Input: dimensioned drawing with shaded views. Units: mm. Origin: part minimum x, y, z. Coordinates: 2 decimals unless noted, no trailing zeros. Order: outer loops, then holes, each group sorted by start corner. A loop starts at its lowest first (then second) coordinate and runs counter-clockwise, first axis right, second up. Notation, with made-up numbers: (21.25, -26) - (47.25, -26) arc R14 ccw to (47.25, -13) - close; hole circle Ø5 at (66.5, 20). An arc over 180 degrees is marked (long way). Answer as CSV lines item,"result". Start each with the question number.
Item 1: Draft query along Y for the marked faces 1, 2 and 3. Return one class per face: +Y half, -Y half, draft (parallel to the pull), parting line (faces both ways), or undercut.
Item 2: First-contact query: pin 1 (1.5 mm diameter, centred on y = 143.5, z = 11.5, fed in from +X); pin 2 (12 mm diameter, centred on x = 36.5, y = 100.5, fed in from +Z); pin 3 (1.5 mm diameter, centred on x = 12.5, z = 12, fed in from -Y). Flat tips, straight axial feed; report the tip coordinate or a pass-through.
Item 3: Section D-D (y = 98). Output: boundary loops of the cut face in (x, z).
Item 4: Section A-A (x = 30). Output: boundary loops of the cut face in (y, z), and give its area (3 significant figures).
Item 5: Section C-C (x = 12.5). Output: boundary loops of the cut face in (y, z).
Item 6: Section B-B (y = 142). Output: boundary loops of the cut face in (x, z).
Item 7: Material intervals for line 1 along X through (y, z) = (142, 5.5); line 2 along Y through (x, z) = (30, 9.5); line 3 along Z through (x, y) = (43, 84), sorted ascending.
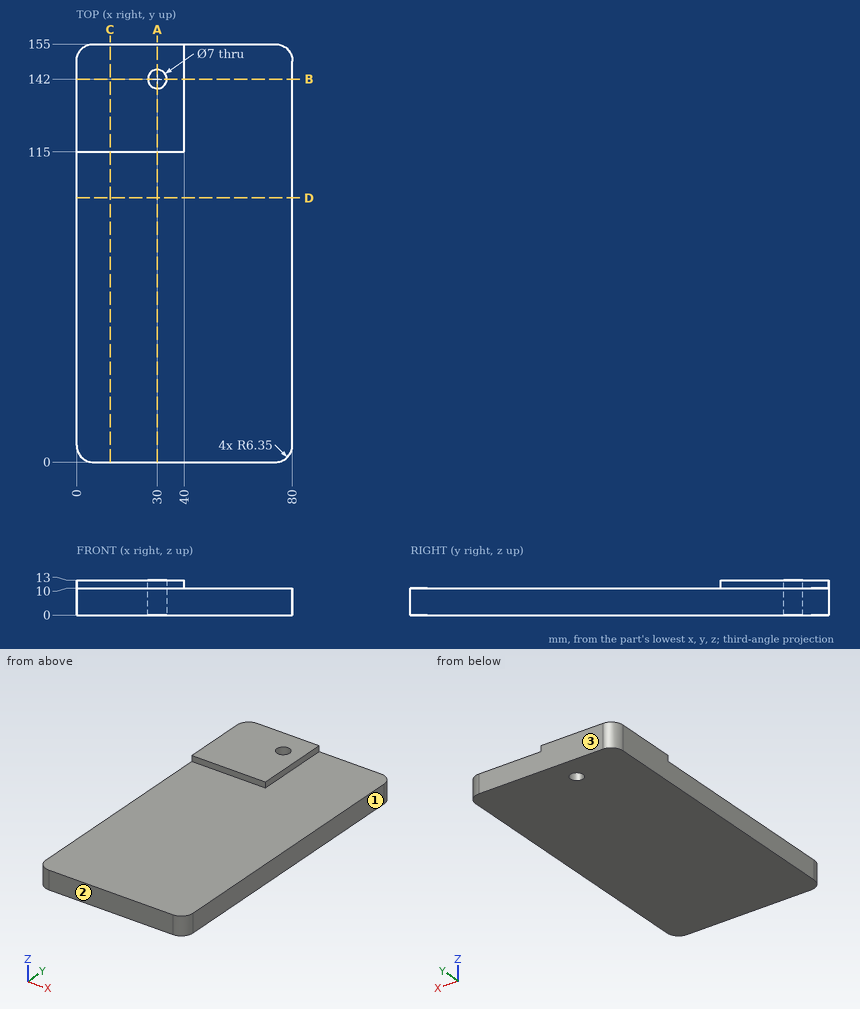
Determined:
1,face 1,"draft"
1,face 2,"-Y half"
1,face 3,"+Y half"
2,pin 1,"stops at x = 40"
2,pin 2,"stops at z = 10"
2,pin 3,"stops at y = 115"
3,outline,"(0, 0) - (80, 0) - (80, 10) - (0, 10) - close"
4,outline,"(0, 0) - (138.5, 0) - (138.5, 13) - (115, 13) - (115, 10) - (0, 10) - close; (145.5, 0) - (155, 0) - (155, 13) - (145.5, 13) - close"
4,area,"1,580 mm^2"
5,outline,"(0, 0) - (155, 0) - (155, 13) - (115, 13) - (115, 10) - (0, 10) - close"
6,outline,"(0, 0) - (26.5, 0) - (26.5, 13) - (0, 13) - close; (33.5, 0) - (80, 0) - (80, 10) - (40, 10) - (40, 13) - (33.5, 13) - close"
7,line 1,"x = 0 to 26.5, 33.5 to 80"
7,line 2,"y = 0 to 138.5, 145.5 to 155"
7,line 3,"z = 0 to 10"
